from build123d import *

# Parameters (mm, degrees)
SKETCH1_W           = 71.12
SKETCH1_H           = 31.5
BOSS_EXTRUDE1_DEPTH = 18.6944
BOSS_EXTRUDE1_TAPER = 10
SKETCH3_R           = 4
CUT_EXTRUDE1_DEPTH  = 2.54
CHAMFER1_SIZE       = 2.54
BOSS_EXTRUDE2_DEPTH = 6.55
BOSS_EXTRUDE3_START = 29.95
BOSS_EXTRUDE3_DEPTH = 29.95


# Some blends are built 0.0001 mm under size
with BuildPart() as part:
    # Sketch1 → Boss-Extrude1 (new body)
    with BuildSketch(Plane(origin=(0, 0, 0), x_dir=(1, 0, 0), z_dir=(0, 1, 0))):
        with Locations((16.51, 0)):
            Rectangle(SKETCH1_W, SKETCH1_H)
    extrude(amount=BOSS_EXTRUDE1_DEPTH, taper=BOSS_EXTRUDE1_TAPER)

    # Fillet1
    # an asymmetric fillet: 16.764, 6.35 mm, written as the material it takes off along each edge
    with BuildSketch(Plane(origin=(59.161619342, -40.218571846, 22.841619342), x_dir=(-0.985255774317392, -0.16848866057223846, 0.029709096802316298), z_dir=(-0.1710878697460354, 0.9702875252478138, -0.17108786974603588))) as fillet1_piece_1:
        with BuildLine():
            Bezier((16.580063455, 0), (0, 0), (-0.17631352, -5.844503547), weights=[1, 0.717688543, 1])
            Line((-0.17631352, -5.844503547), (0, 0))
            Line((0, 0), (16.580063455, 0))
        make_face()
    extrude(amount=102.167183553, mode=Mode.SUBTRACT)
    with BuildSketch(Plane(origin=(-26.141619342, -40.218571846, -22.841619342), x_dir=(-0.029709096802316662, -0.16848866057223877, 0.9852557743173919), z_dir=(0.1710878697460356, 0.9702875252478138, 0.1710878697460358))) as fillet1_piece_2:
        with BuildLine():
            Bezier((5.847162404, 0), (0, 0), (-0.499950087, 16.572524071), weights=[1, 0.717688543, 1])
            Line((-0.499950087, 16.572524071), (0, 0))
            Line((0, 0), (5.847162404, 0))
        make_face()
    extrude(amount=102.167183553, mode=Mode.SUBTRACT)
    with BuildSketch(Plane(origin=(59.161619342, -40.218571846, -22.841619342), x_dir=(0.029709096802316877, -0.16848866057223874, 0.9852557743173919), z_dir=(-0.1710878697460358, 0.9702875252478138, 0.1710878697460358)), Plane(origin=(-26.141619342, -40.218571846, 22.841619342), x_dir=(-0.029709096802316284, -0.16848866057223885, -0.9852557743173919), z_dir=(0.1710878697460356, 0.9702875252478138, -0.1710878697460358))) as fillet1_piece_3:
        with BuildLine():
            Bezier((5.847162404, 0), (0, 0), (-0.499950087, -16.572524071), weights=[1, 0.717688543, 1])
            Line((-0.499950087, -16.572524071), (0, 0))
            Line((0, 0), (5.847162404, 0))
        make_face()
    extrude(amount=102.167183553, mode=Mode.SUBTRACT)

    # Sketch3 → Cut-Extrude1 (cut)
    with BuildSketch(Plane.XZ):
        with Locations(Location((0, 0, 0), (0, 0, 270))):
            Circle(SKETCH3_R)
    extrude(amount=-CUT_EXTRUDE1_DEPTH, mode=Mode.SUBTRACT)

    # Chamfer1
    chamfer1_edges = [part.edges().sort_by_distance(p)[0] for p in [
        (0, 0, 4),
    ]]
    chamfer(chamfer1_edges, length=CHAMFER1_SIZE - 0.0001)  # a hair under: the kernel refuses the full size

    # Sketch4 → Boss-Extrude2 (add)
    with BuildSketch(Plane(origin=(0, 0, 0), x_dir=(0, 0, -1), z_dir=(1, 0, 0))):
        with BuildLine():
            Line((30.48, 64.4144), (30.48, 72.0344))
            Line((30.48, 72.0344), (-3.81, 72.0344))
            ThreePointArc((-3.81, 72.0344), (-6.504076836, 70.918476836), (-7.62, 68.2244))
            Line((-7.62, 68.2244), (-7.62, 64.4144))
            Line((-7.62, 64.4144), (-7.62, 28.0924))
            ThreePointArc((-7.62, 28.0924), (-6.504076836, 25.398323164), (-3.81, 24.2824))
            Line((-3.81, 24.2824), (-2.756322634, 24.2824))
            Line((-2.756322634, 24.2824), (-2.756322634, 18.6944))
            Line((-2.756322634, 18.6944), (2.756322634, 18.6944))
            Line((2.756322634, 18.6944), (2.756322634, 24.2824))
            Line((2.756322634, 24.2824), (10.668, 24.2824))
            Line((10.668, 24.2824), (10.668, 26.3144))
            Line((10.668, 26.3144), (0, 26.3144))
            Line((0, 26.3144), (0, 64.4144))
            Line((0, 64.4144), (30.48, 64.4144))
        make_face()
    extrude(amount=-BOSS_EXTRUDE2_DEPTH)

    # Sketch5 → Boss-Extrude3 (add)
    with BuildSketch(Plane(origin=(0, 0, 0), x_dir=(0, 0, -1), z_dir=(1, 0, 0)).offset(BOSS_EXTRUDE3_START)):
        with BuildLine():
            Line((-7.62, 68.2244), (-7.62, 28.0924))
            ThreePointArc((-7.62, 28.0924), (-6.504076836, 25.398323164), (-3.81, 24.2824))
            Line((-3.81, 24.2824), (-2.756322634, 24.2824))
            Line((-2.756322634, 24.2824), (-2.756322634, 18.6944))
            Line((-2.756322634, 18.6944), (2.756322634, 18.6944))
            Line((2.756322634, 18.6944), (2.756322634, 24.2824))
            Line((2.756322634, 24.2824), (10.668, 24.2824))
            Line((10.668, 24.2824), (10.668, 26.3144))
            Line((10.668, 26.3144), (0, 26.3144))
            Line((0, 26.3144), (0, 64.4144))
            Line((0, 64.4144), (30.48, 64.4144))
            Line((30.48, 64.4144), (30.48, 72.0344))
            Line((30.48, 72.0344), (-3.81, 72.0344))
            ThreePointArc((-3.81, 72.0344), (-6.504076836, 70.918476836), (-7.62, 68.2244))
        make_face()
    extrude(amount=-BOSS_EXTRUDE3_DEPTH)


solid = part.part
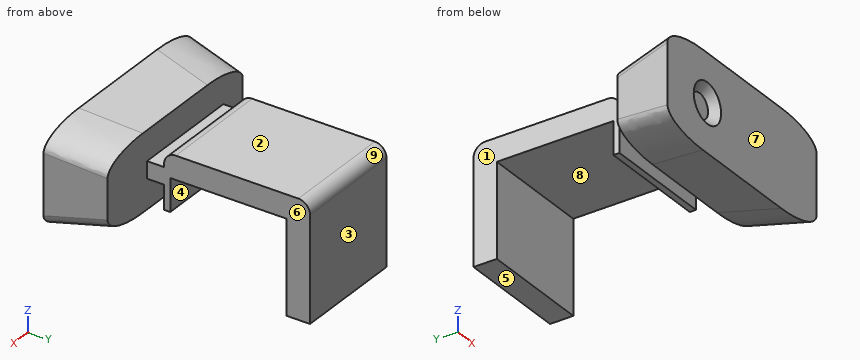
Here's how the part is built. I have some questions about the finished solid (model axes, mm). Face numbers are marked on the shaded views. A direction names the side the tool comes from. Coordinates: 2 decimals unless noted, no trailing zeros. Order: outer loops, then holes, each group sorted by start corner. A loop starts at its lowest first (then second) coordinate and runs counter-clockwise, first axis right, second up. Notation, with made-up numbers: (25.25, -4) - (79.25, -4) arc R12 cw to (79.25, 0) - close; hole circle Ø1 at (-40, -18). An arc over 180 degrees is marked (long way). Use CSV: the item, a comma, the result in double quotes. Start each with the question number.
1. If we mould it in two halves opening along Y, with no side actions, what happens to the marked faces 6, 7, 8 and 9? For each: +Y half, -Y half, draft (parallel to the pull), parting line (faces both ways), or undercut.
2. I'm going to push flat-ended pins straight in: pin 1 (19 mm diameter, centred on y = 52.5, z = -3.5, fed in from +X); pin 2 (6 mm diameter, centred on x = 13, y = 22.5, fed in from +Z); pin 3 (8 mm diameter, centred on x = 36.5, y = 11, fed in from +Z). Where does each tip first touch, or does it pass through?
3. Suppose I cut it at A-A on y = 22. List the corners of the cut face in (x, z) for me, then the cut area to 3 significant figures.
4. For the marked faces 1, 2, 3, 4 and 5, which set-ups out of +Z, -Z, +X, -X, +Y, -Y let a thin tool reach every point of the face, with its end or its side?
5. Suppose I cut it at B-B on z = -27. List the corners of the cut face in (x, y) for me, then the cut area to 3 significant figures.
6. Please list where these lines run through material, in increasing order: line 1 (Y direction, x = 22.5, z = -7.5); line 2 (Y direction, x = 24.5, z = -17); line 3 (Z direction, x = 0, y = 2). Write a range as from..to.
Output:
1,face 6,"draft"
1,face 7,"-Y half"
1,face 8,"undercut"
1,face 9,"+Y half"
2,pin 1,"stops at x = 29.95"
2,pin 2,"stops at z = 6.6"
2,pin 3,"stops at z = 14.47"
3,outline,"(-6.55, -2.76) - (29.95, -2.76) - (29.95, 2.76) - (-6.55, 2.76) - close"
3,area,"201 mm2"
4,face 1,"+Z, -Z, -X, +Y"
4,face 2,"+Z, +X, -X, +Y"
4,face 3,"+Z, -Z, +X, -X, +Y"
4,face 4,"-Z, +X, -X"
4,face 5,"-Z, +X, -X, +Y, -Y"
5,outline,"(-6.55, 64.41) - (29.95, 64.41) - (29.95, 72.03) - (-6.55, 72.03) - close"
5,area,"278 mm2"
6,line 1,"y = 0..18.69, 24.28..26.31, 64.41..72.03"
6,line 2,"y = 64.41..72.03"
6,line 3,"z = -15.4..-4.54, 4.54..15.4"
